```python
from build123d import *

# Parameters (mm, degrees)
RESSALTO_EXTRUS_O1_DEPTH = 5
ESBO_O2_R                = 1.5
CORTE_EXTRUS_O1_DEPTH    = 10
ESBO_O3_R                = 1.5
CORTE_EXTRUS_O2_DEPTH    = 6


with BuildPart() as part:
    # Esboço1 → Ressalto-extrusão1 (new body)
    with BuildSketch(Plane.XY):
        Polygon((-1.556986729, 38.142857143), (16.443013271, 38.142857143), (16.443013271, 46.142857143), (36.443013271, 46.142857143), (36.443013271, 38.142857143), (42.443013271, 38.142857143), (42.443013271, -34.857142857), (-27.556986729, -34.857142857), (-27.556986729, 38.142857143), (-21.556986729, 38.142857143), (-21.556986729, 46.142857143), (-1.556986729, 46.142857143), align=None)
    extrude(amount=RESSALTO_EXTRUS_O1_DEPTH)

    # Esboço2 → Corte-extrusão1 (cut)
    with BuildSketch(Plane.XY.offset(5)):
        with Locations((-17.556986729, 43.142857143)):
            Circle(ESBO_O2_R)
        with Locations((-6.556986729, 43.142857143)):
            Circle(ESBO_O2_R)
    extrude(amount=-CORTE_EXTRUS_O1_DEPTH, mode=Mode.SUBTRACT)

    # Esboço3 → Corte-extrusão2 (cut, through all)
    with BuildSketch(Plane.XY.offset(5)):
        with Locations((21.443013271, 43.142857143)):
            Circle(ESBO_O3_R)
        with Locations((31.443013271, 43.142857143)):
            Circle(ESBO_O3_R)
    extrude(amount=-CORTE_EXTRUS_O2_DEPTH, mode=Mode.SUBTRACT)


solid = part.part
```
Part model, mm, in its own coordinate system. A direction names the side the tool comes from. Round coordinates to 2 decimals unless told otherwise and drop trailing zeros. Write each loop counter-clockwise with the first axis right and the second up, starting at its lowest first coordinate (ties: lowest second). Pieces come first, ordered by that corner, then holes.
Item 1: Drop flat-ended pins along their axis: pin 1 Ø2.5 at (x, y) = (21.44, 43.14) entering from -Z; pin 2 Ø1.5 at (y, z) = (40.5, 3) entering from -X; pin 3 Ø1.5 at (y, z) = (42.5, 2) entering from +X. Give the stop position or say it passes through.
Results:
pin 1: passes through
pin 2: stops at x = -21.56
pin 3: stops at x = 36.44
Item 2: Cut at C-C, the plane x = 9. Give the cut face in (y, z), plus the area to 3 significant figures.
Results:
outline: (-34.86, 0) - (38.14, 0) - (38.14, 5) - (-34.86, 5) - close
area: 365 mm2
Item 3: Which spindle directions (+Z, -Z, +X, -X, +Y, -Y) get a long thin tool onto all of the face, cutting with end or side? Do faces 5 (the flat face through (-25, 38.143, 2)), 6 (the flat face through (36.443, 42, 2)), 7 (the flat face through (16.443, 42, 2)). Say none if no direction does.
Results:
face 5: +Z, -Z, -X, +Y
face 6: +Z, -Z, +X, +Y
face 7: +Z, -Z, +Y
Item 4: Cut at B-B, the plane x = -17.5. Give the cut face in (y, z).
Results:
outline: (-34.86, 0) - (41.64, 0) - (41.64, 5) - (-34.86, 5) - close; (44.64, 0) - (46.14, 0) - (46.14, 5) - (44.64, 5) - close
Item 5: Cut at A-A, the plane z = 2.9. Give the cut face in (x, y), plus the area to 3 significant figures.
Results:
outline: (-27.56, -34.86) - (42.44, -34.86) - (42.44, 38.14) - (36.44, 38.14) - (36.44, 46.14) - (16.44, 46.14) - (16.44, 38.14) - (-1.56, 38.14) - (-1.56, 46.14) - (-21.56, 46.14) - (-21.56, 38.14) - (-27.56, 38.14) - close; hole circle Ø3 at (-17.56, 43.14); hole circle Ø3 at (-6.56, 43.14); hole circle Ø3 at (21.44, 43.14); hole circle Ø3 at (31.44, 43.14)
area: 5,400 mm2
Item 6: Two-plate mould, pull along Y, no slides. Class faces 1 (the flat face through (-21.557, 42, 2)), 2 (the flat face through (26, 46.143, 2)), 3 (the cylindrical face through (30.253, 42.23, 2.535)), 4 (the flat face through (8, -34.857, 2)): +Y half, -Y half, draft (parallel to the pull), parting line (faces both ways), or undercut.
Results:
face 1: draft
face 2: +Y half
face 3: undercut
face 4: -Y half
Item 7: Probe L1, parallel to Y at x = -6.5, z = 4.5; L2, parallel to Y at x = -0.5, z = 1.15; L3, parallel to X at y = 41, z = 2.7. List the from-to ranges inside material, lowest first.
Results:
L1: y = -34.86 to 41.64, 44.64 to 46.14
L2: y = -34.86 to 38.14
L3: x = -21.56 to -1.56, 16.44 to 36.44
Item 8: Cut at D-D, the plane x = 31. Give the cut face in (y, z).
Results:
outline: (-34.86, 0) - (41.71, 0) - (41.71, 5) - (-34.86, 5) - close; (44.58, 0) - (46.14, 0) - (46.14, 5) - (44.58, 5) - close
